Model file for the job. Use its own axes, mm. A direction names the side the tool comes from. Coordinates: 2 decimals unless noted, no trailing zeros. Write each loop counter-clockwise with the first axis right and the second up, starting at its lowest first coordinate (ties: lowest second). Pieces come first, ordered by that corner, then holes.
Q1. Pull direction Z, two halves, no side cores. Call faces 1 (the cylindrical face through (6.97, 2.197, -9.245)), 2 (the flat face through (18, 2.4, -2)), 3 (the flat face through (10.313, 2.197, -4.913)): released by +Z, released by -Z, zero draft, split by the parting line, or undercut.
Q2. Which spindle directions (+Z, -Z, +X, -X, +Y, -Y) get a long thin tool onto all of the face, cutting with end or side? Do faces 4 (the flat face through (10, 1, -10)), 5 (the flat face through (1.5, 2.4, -1.5)), 6 (the cylindrical face through (19.803, 1.15, -7.977)), 7 (the flat face through (6, 2.4, -6)), 8 (the cylindrical face through (19.21, 2.2, -2.13)). Say none if no direction does.
Q3. Band-saw the part on D-D, the plane z = -1.5. Write the cut outline in (x, y).
Q4. Band-saw the part on C-C, the plane x = 18.5. Write the cut outline in (y, z), plus the area to 3 significant figures.
Q5. Band-saw the part on B-B, the plane y = 1.2. Write the cut outline in (x, z), plus the area to 3 significant figures.
Q6. Drill centre lines: probe 1 along X at (y, z) = (0.75, -5); probe 2 along Y at (x, z) = (19.7, -5.5); probe 3 along X at (y, z) = (2.25, -5). Where is each one in solid material? Low to high.
Q7. Pin check, flat tips, straight feed: P1, Ø3, axis at x = 2, z = -5, coming from the +Y side; P2, Ø1.8, axis at x = 12, z = -5.5, coming from the +Y side; P3, Ø0.8, axis at y = 1, z = -5.5, coming from the +X side. Stop position of each tip, or through.
Q8. Band-saw the part on A-A, the plane x = 2. Write the cut outline in (y, z), plus the area to 3 significant figures.
from build123d import *

# Parameters (mm, degrees)
SKETCH1_W           = 20
SKETCH1_H           = 10
SKETCH1_R           = 1
BOSS_EXTRUDE1_DEPTH = 2
SKETCH2_W           = 0.628205128
SKETCH2_H           = 3.5
BOSS_EXTRUDE2_DEPTH = 0.4
SKETCH4_W           = 8
SKETCH4_H           = 0.4
CUT_EXTRUDE4_DEPTH  = 0.4
SKETCH5_R           = 0.8
BOSS_EXTRUDE3_DEPTH = 0.4
SKETCH7_R           = 0.581669736
BOSS_EXTRUDE4_DEPTH = 0.4
SKETCH6_R           = 0.420338274
BOSS_EXTRUDE5_DEPTH = 0.4
CIRPATTERN1_COUNT   = 6
SKETCH8_R           = 0.5
CUT_EXTRUDE6_DEPTH  = 0.4
LPATTERN1_COUNT     = 4
LPATTERN1_PITCH     = 2
BOSS_EXTRUDE6_START = -2
SKETCH10_R          = 1
BOSS_EXTRUDE6_DEPTH = 0.4


with BuildPart() as part:
    # Sketch1 → Boss-Extrude1 (new body)
    with BuildSketch(Plane(origin=(0, 0, 0), x_dir=(1, 0, 0), z_dir=(0, 1, 0))):
        with Locations((10, 5)):
            Rectangle(SKETCH1_W, SKETCH1_H)
        with Locations(Location((2, 5, 0), (0, 0, 270))):
            Circle(SKETCH1_R, mode=Mode.SUBTRACT)
    extrude(amount=BOSS_EXTRUDE1_DEPTH)

    # Sketch2 → Boss-Extrude2 (add)
    # profile 1 of 3: a face of its own
    with BuildSketch(Plane(origin=(0, 2, 0), x_dir=(1, 0, 0), z_dir=(0, 1, 0))):
        Polygon((9.033403528, 6.638234894), (9.616035739, 6.638234894), (11.029497278, 3.138234894), (10.35852372, 3.138234894), (10.086488463, 3.856183612), (8.56154856, 3.856183612), (8.289513303, 3.138234894), (7.619240867, 3.138234894), align=None)
        Polygon((9.324369072, 5.69943281), (8.79992997, 4.48438874), (9.848808175, 4.48438874), align=None, mode=Mode.SUBTRACT)
    # profile 2 of 3: a face of its own
    with BuildSketch(Plane(origin=(0, 2, 0), x_dir=(1, 0, 0), z_dir=(0, 1, 0))):
        Polygon((11.545522919, 6.638234894), (12.173728047, 6.638234894), (12.173728047, 3.766440022), (13.160907534, 3.766440022), (13.160907534, 3.138234894), (11.545522919, 3.138234894), align=None)
    # profile 3 of 3: a face of its own
    with BuildSketch(Plane(origin=(0, 2, 0), x_dir=(1, 0, 0), z_dir=(0, 1, 0))):
        with Locations((13.923728047, 4.888234894)):
            Rectangle(SKETCH2_W, SKETCH2_H)
    extrude(amount=BOSS_EXTRUDE2_DEPTH)

    # Sketch4 → Cut-Extrude4 (cut)
    with BuildSketch(Plane(origin=(0, 2, 0), x_dir=(1, 0, 0), z_dir=(0, 1, 0))):
        with Locations((11.161065363, 2.289063397)):
            Rectangle(SKETCH4_W, SKETCH4_H)
    extrude(amount=-CUT_EXTRUDE4_DEPTH, mode=Mode.SUBTRACT)

    # Sketch5 → Boss-Extrude3 (add)
    with BuildSketch(Plane(origin=(0, 2, 0), x_dir=(1, 0, 0), z_dir=(0, 1, 0))):
        with Locations(Location((1.5, 8.5, 0), (0, 0, 90))):
            Circle(SKETCH5_R)
        with Locations(Location((18.5, 8.630956257, 0), (0, 0, 90))):
            Circle(SKETCH5_R)
        with Locations(Location((18.5, 1.759911555, 0), (0, 0, 90))):
            Circle(SKETCH5_R)
        with Locations(Location((1.5, 1.5, 0), (0, 0, 90))):
            Circle(SKETCH5_R)
    extrude(amount=BOSS_EXTRUDE3_DEPTH)

    # Sketch7 → Boss-Extrude4 (add)
    with BuildSketch(Plane(origin=(0, 2, 0), x_dir=(1, 0, 0), z_dir=(0, 1, 0))):
        with Locations(Location((7.145081421, 8.690538135, 0), (0, 0, 90))):
            Circle(SKETCH7_R)
    boss_extrude4 = extrude(amount=BOSS_EXTRUDE4_DEPTH)

    # Sketch6 → Boss-Extrude5 (add)
    with BuildSketch(Plane(origin=(0, 2, 0), x_dir=(1, 0, 0), z_dir=(0, 1, 0))):
        with Locations(Location((5.883797923, 7.542946747, 0), (0, 0, 90))):
            Circle(SKETCH6_R)
    extrude(amount=BOSS_EXTRUDE5_DEPTH)

    # CirPattern1: Boss-Extrude4 ×6 about axis
    cirpattern1_axis = Axis((5.883797923, 0, -7.542946747), (0, 1, 0))
    for i in range(1, CIRPATTERN1_COUNT):
        add(boss_extrude4.rotate(cirpattern1_axis, i * 360 / CIRPATTERN1_COUNT))

    # Sketch8 → Cut-Extrude6 (cut)
    with BuildSketch(Plane(origin=(20, 0, 0), x_dir=(0, 0, -1), z_dir=(1, 0, 0))):
        with Locations((1.5, 1)):
            Circle(SKETCH8_R)
    cut_extrude6 = extrude(amount=-CUT_EXTRUDE6_DEPTH, mode=Mode.SUBTRACT)

    # LPattern1: Cut-Extrude6 ×4
    with Locations(*[(0, 0, -i * LPATTERN1_PITCH) for i in range(1, LPATTERN1_COUNT)]):
        add(cut_extrude6, mode=Mode.SUBTRACT)

    # Sketch10 → Boss-Extrude6 (add)
    with BuildSketch(Plane.XY.offset(BOSS_EXTRUDE6_START)):
        with Locations((5.5, 1.5)):
            Circle(SKETCH10_R)
    extrude(amount=-BOSS_EXTRUDE6_DEPTH)


solid = part.part
Answer sheet:
1. face 1: undercut
1. face 2: zero draft
1. face 3: released by -Z
2. face 4: -Z, +X, -X, +Y, -Y
2. face 5: +Z, -Z, -X, +Y
2. face 6: +X
2. face 7: -Z, +X, -X, +Y
2. face 8: +Y
3. outline: (0, 0) - (20, 0) - (20, 0.5) - (19.6, 0.5) - (19.6, 1.5) - (20, 1.5) - (20, 2) - (19.26, 2) - (19.26, 2.4) - (17.74, 2.4) - (17.74, 2) - (2.3, 2) - (2.3, 2.4) - (0.7, 2.4) - (0.7, 2) - (0, 2) - close
4. outline: (0, -10) - (2, -10) - (2, -9.43) - (2.4, -9.43) - (2.4, -7.83) - (2, -7.83) - (2, -2.56) - (2.4, -2.56) - (2.4, -0.96) - (2, -0.96) - (2, 0) - (0, 0) - close
4. area: 21.3 mm2
5. outline: (0, -10) - (20, -10) - (20, -7.96) - (19.6, -7.96) - (19.6, -7.04) - (20, -7.04) - (20, -5.96) - (19.6, -5.96) - (19.6, -5.04) - (20, -5.04) - (20, -3.96) - (19.6, -3.96) - (19.6, -3.04) - (20, -3.04) - (20, -1.96) - (19.6, -1.96) - (19.6, -1.04) - (20, -1.04) - (20, 0) - (0, 0) - close; hole circle Ø2 at (2, -5)
5. area: 195 mm2
6. probe 1: x = 0 to 1, 3 to 20
6. probe 2: y = 0 to 0.5, 1.5 to 2
6. probe 3: x = 8.37 to 9.02, 9.63 to 10.28, 11.55 to 12.17, 13.61 to 14.24
7. P1: stops at y = 2
7. P2: stops at y = 2.4
7. P3: stops at x = 19.6
8. outline: (0, -10) - (2, -10) - (2, -9.12) - (2.4, -9.12) - (2.4, -7.88) - (2, -7.88) - (2, -6) - (0, -6) - close; (0, -4) - (2, -4) - (2, -2.12) - (2.4, -2.12) - (2.4, -0.88) - (2, -0.88) - (2, 0) - (0, 0) - close
8. area: 17.0 mm2
